Could you check a few things on this drawing? It's one solid part, dimensions in mm from its lowest x, y, z. Give positions to 0.01 mm unless a question says otherwise; leave off trailing zeros. Loops run counter-clockwise (first coordinate to the right, second up) from the corner with the lowest first, then second, coordinate; pieces in that order, holes last. Notation, with made-up numbers: (-20, 67) - (-9, 67) arc R23 ccw to (-9, 91) - close; hole circle Ø6 at (65, 33.25). An arc over 180 degrees is marked (long way). Put each result on its own line as item: value. Start each with the question number.
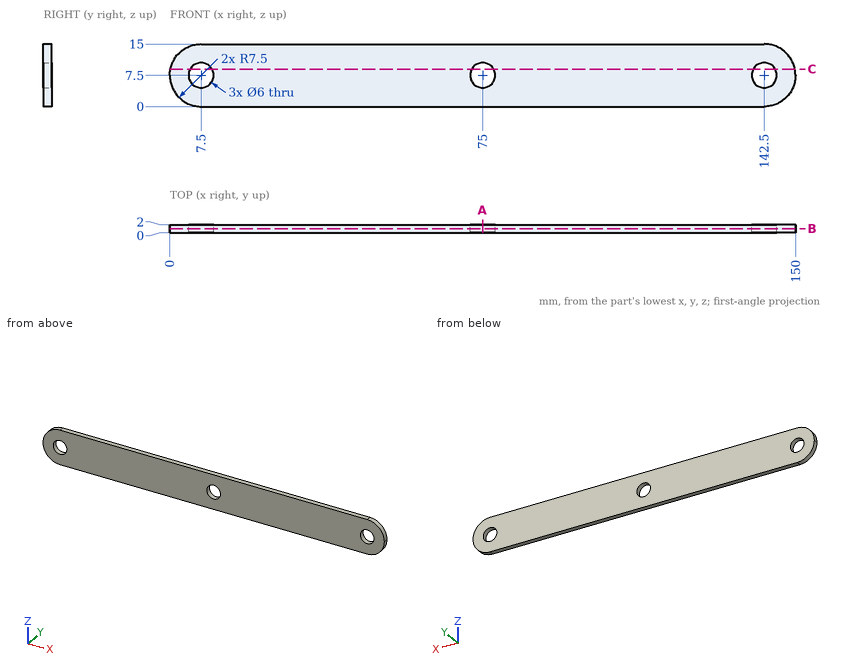
1) Suppose I cut it at C-C on z = 9. Please give me the cut outline in (x, y), plus the area to 3 significant figures.
2) I'm going to push a flat-ended pin straight in: P1, Ø8, axis at x = 31, z = 7, coming from the -Y side. Where does the tip first touch, or does it pass through?
3) I need wall thicknesses on line 1 (Z direction, x = 75, y = 1.6); line 2 (X direction, y = 1.9, z = 5.25); line 3 (X direction, y = 0.85, z = 6.25). Which ranges of each line are inside material? Lowest first, please.
4) Suppose I cut it at B-B on y = 1.05. Give the number of separate pieces and of enclosed holes in the cut face, plus the area to 3 significant figures.
5) Suppose I cut it at A-A on x = 75. Please give me the cut outline in (y, z), plus the area to 3 significant figures.
Ans:
1. outline: (0.15, 0) - (4.9, 0) - (4.9, 2) - (0.15, 2) - close; (10.1, 0) - (72.4, 0) - (72.4, 2) - (10.1, 2) - close; (77.6, 0) - (139.9, 0) - (139.9, 2) - (77.6, 2) - close; (145.1, 0) - (149.85, 0) - (149.85, 2) - (145.1, 2) - close
1. area: 268 mm²
2. P1: stops at y = 0
3. line 1: z = 0 to 4.5, 10.5 to 15
3. line 2: x = 0.35 to 5.52, 9.48 to 73.02, 76.98 to 140.52, 144.48 to 149.65
3. line 3: x = 0.1 to 4.77, 10.23 to 72.27, 77.73 to 139.77, 145.23 to 149.9
4. separate pieces: 1
4. enclosed holes: 3
4. area: 2,120 mm²
5. outline: (0, 0) - (2, 0) - (2, 4.5) - (0, 4.5) - close; (0, 10.5) - (2, 10.5) - (2, 15) - (0, 15) - close
5. area: 18.0 mm²
